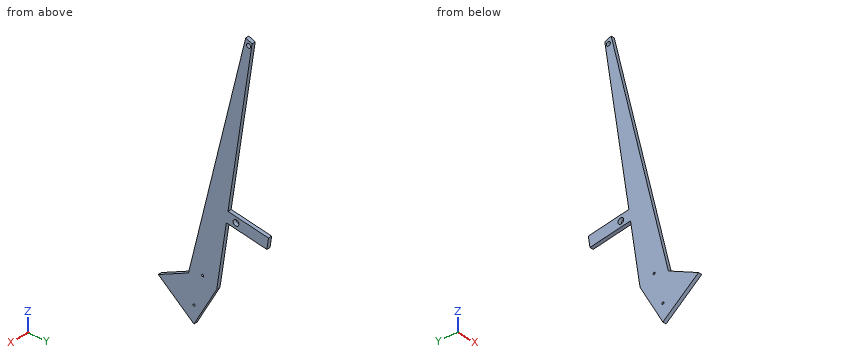
```python
from build123d import *

# Parameters (mm, degrees)
SKETCH_1_R          = 0.6
SKETCH_1_R_2        = 1.16208208
EXTRUDE_1_DEPTH     = 2
SKETCH_2_W          = 2
SKETCH_2_H          = 6.221940724
EXTRUDE_2_DEPTH     = 22.998818
SKETCH_3_R          = 1.614508757
CUT_EXTRUDE_1_DEPTH = 136.634989839


with BuildPart() as part:
    # 草图1 → 凸台-拉伸1 (new body)
    with BuildSketch(Plane(origin=(0, 0, 0), x_dir=(0, 0, -1), z_dir=(1, 0, 0))):
        Polygon((-129.110885337, 27.705001714), (3.4977294, 7.905798819), (26.635169992, -4.901598114), (10.519539729, -24.901019931), (2.231501308, -7.979608155), (-130.492225074, 24.136540727), align=None)
        Circle(SKETCH_1_R, mode=Mode.SUBTRACT)
        with Locations((17.069222108, -4.901598114)):
            Circle(SKETCH_1_R, mode=Mode.SUBTRACT)
        with Locations((-127.222518318, 25.717836253)):
            Circle(SKETCH_1_R_2, mode=Mode.SUBTRACT)
    extrude(amount=EXTRUDE_1_DEPTH)

    # 草图2 → 凸台-拉伸2 (add)
    with BuildSketch(Plane(origin=(0, 8.244247262, -1.230911918), x_dir=(1, 0, 0), z_dir=(0, 0.9890368823707517, -0.14766870118729958))):
        with Locations((1, -37.181709338)):
            Rectangle(SKETCH_2_W, SKETCH_2_H)
    extrude(amount=EXTRUDE_2_DEPTH)

    # 草图3 → 切除-拉伸1 (cut, through all)
    with BuildSketch(Plane(origin=(2, 0, 0), x_dir=(0, 0, -1), z_dir=(1, 0, 0))):
        with Locations((-34.804826462, 18.6800064)):
            Circle(SKETCH_3_R)
    extrude(amount=-CUT_EXTRUDE_1_DEPTH, mode=Mode.SUBTRACT)


solid = part.part
```
Work out the finished part from the listing and answer in its coordinate system (mm). Round coordinates to 2 decimals unless told otherwise and drop trailing zeros. Loops run counter-clockwise (first coordinate to the right, second up) from the corner with the lowest first, then second, coordinate; pieces in that order, holes last.
(1) Find the intervals of material crossed by L1, parallel to Y at x = 0.3, z = 35; L2, parallel to Z at x = 1.5, y = -8; L3, parallel to Y at x = 1, z = 24, in increasing order.
Computed values:
L1: y = 1.03 to 17.08, 20.28 to 36.91
L2: z = -24.14 to -2.24
L3: y = -1.63 to 12.01
(2) The part is cut by section B-B, the plane z = 78. Give the vertices of the cut face in (x, y), and give its area (3 significant figures).
Computed values:
outline: (0, 11.43) - (2, 11.43) - (2, 20.07) - (0, 20.07) - close
area: 17.3 mm2
(3) The part is cut by section A-A, the plane x = 1.2. Give the vertices of the cut face in (y, z) (1 decimal).
Computed values:
outline: (-24.9, -10.5) - (-4.9, -26.6) - (7.9, -3.5) - (13.3, 32.5) - (36, 29.1) - (36.9, 35.2) - (14.2, 38.6) - (27.7, 129.1) - (24.1, 130.5) - (-8, -2.2) - close; hole circle Ø1.2 at (-4.9, -17.1); hole circle Ø1.2 at (0, 0); hole circle Ø3.2 at (18.7, 34.8); hole circle Ø2.3 at (25.7, 127.2)
(4) This flat-tipped pin is pushed along its axis until it touches: P1, Ø4, axis at y = 18.68, z = 34.8, coming from the +X side. Where does it stop, or does it pass through?
Computed values:
P1: stops at x = 2
(5) The part is cut by section C-C, the plane y = 31. Give the vertices of the cut face in (x, z), and give its area (3 significant figures).
Computed values:
outline: (0, 29.82) - (2, 29.82) - (2, 36.11) - (0, 36.11) - close
area: 12.6 mm2
